Work out the finished part from the listing and answer in its coordinate system (mm). Coordinates: 2 decimals unless noted, no trailing zeros. Order: outer loops, then holes, each group sorted by start corner. A loop starts at its lowest first (then second) coordinate and runs counter-clockwise, first axis right, second up.
1. The part is cut by section A-A, the plane z = 12.7. Give the vertices of the cut face in (x, y).
2. The part is cut by section B-B, the plane z = 0. Give the vertices of the cut face in (x, y), then the cut area to 3 significant figures.
3. Flat-ended cylindrical pins translate along their axes: pin 1 Ø0.6 at (x, y) = (-33, 3) entering from +Z; pin 2 Ø2 at (y, z) = (3.5, 39.5) entering from -X; pin 3 Ø1.5 at (x, y) = (-41, 3.5) entering from -Z. Find the tip coordinate at first contact, or state that the pin passes through.
4. The part is cut by section D-D, the plane y = 3.25. Count the separate pieces of the cut face and the enclosed holes in it, then the cut area to 3 significant figures.
5. The part is cut by section C-C, the plane z = 51. Give the vertices of the cut face in (x, y).
6. Find the intervals of material crossed by probe 1 along X at (y, z) = (0.5, 0.5); probe 2 along Z at (x, y) = (-32, 5); probe 3 along Z at (x, y) = (-20.5, 2.75) (3 decimals), in increasing order.
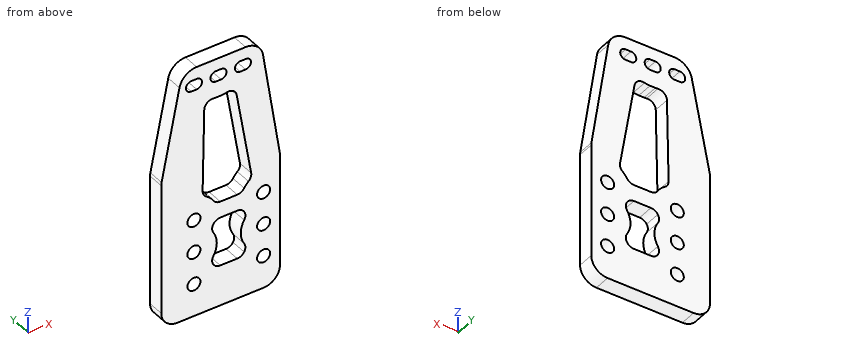
Autodesk Inventor part; units mm, degrees
ref_plane "YZ Plane" through (0, 0, 0) normal (1, 0, 0) x (0, 1, 0)
ref_plane "XZ Plane" through (0, 0, 0) normal (0, 1, 0) x (-1, 0, 0)
ref_plane "XY Plane" through (0, 0, 0) normal (0, 0, 1) x (1, 0, 0)
sketch "Sketch1" plane through (0, 0, 0) normal (0, 1, 0) x (-1, 0, 0)
  line L0 (0, 25.4) -> (0, -25.4) construction
  line L1 (0, -25.4) -> (46.1518, -25.4) construction
  line L2 (15.4178, 64.3509) -> (13.335, 64.3509)
  line L3 (15.4178, 68.5165) -> (13.335, 68.5165)
  arc A0 (13.335, 68.5165) -> (13.335, 64.3509) centre (13.335, 66.4337) ccw
  arc A1 (15.4178, 64.3509) -> (15.4178, 68.5165) centre (15.4178, 66.4337) ccw
  circle A2 centre (13.335, 66.4337) radius 6.8266 construction
  line L4 (32.385, 73.2603) -> (13.335, 73.2603)
  circle A3 centre (6.35, 0) radius 2.54
  circle A4 centre (6.35, -12.7) radius 2.54
  circle A5 centre (6.35, 12.7) radius 2.54
  line L5 (6.35, -12.7) -> (6.35, 12.7) construction
  line L6 (6.5905, 67.4898) -> (0.0764, 25.8882)
  line L7 (0, 24.9059) -> (0, -19.05)
  arc A6 (0.0764, 25.8882) -> (0, 24.9059) centre (6.35, 24.9059) ccw
  line L8 (46.1518, -19.05) -> (46.1518, 31.75)
  line L9 (39.0793, 67.7714) -> (46.0287, 32.9943)
  arc A7 (46.1518, 31.75) -> (46.0287, 32.9943) centre (39.8018, 31.75) ccw
  arc A8 (13.335, 73.2603) -> (6.5905, 67.4898) centre (13.335, 66.4337) ccw
  line L10 (39.8018, -25.4) -> (6.35, -25.4)
  circle A9 centre (33.4518, 12.7) radius 2.54
  circle A10 centre (33.4518, 0) radius 2.54
  circle A11 centre (33.4518, -12.7) radius 2.54
  line L11 (33.4518, -12.7) -> (33.4518, 12.7) construction
  arc A12 (39.8018, -25.4) -> (46.1518, -19.05) centre (39.8018, -19.05) ccw
  arc A13 (0, -19.05) -> (6.35, -25.4) centre (6.35, -19.05) ccw
  arc A14 (24.9428, 64.3509) -> (24.9428, 68.5165) centre (24.9428, 66.4337) ccw
  line L12 (24.9428, 64.3509) -> (22.86, 64.3509)
  line L13 (24.9428, 68.5165) -> (22.86, 68.5165)
  arc A15 (22.86, 68.5165) -> (22.86, 64.3509) centre (22.86, 66.4337) ccw
  circle A16 centre (22.86, 66.4337) radius 6.8266 construction
  arc A17 (34.4678, 64.3509) -> (34.4678, 68.5165) centre (34.4678, 66.4337) ccw
  line L14 (34.4678, 64.3509) -> (32.385, 64.3509)
  line L15 (34.4678, 68.5165) -> (32.385, 68.5165)
  arc A18 (32.385, 68.5165) -> (32.385, 64.3509) centre (32.385, 66.4337) ccw
  circle A19 centre (32.385, 66.4337) radius 6.8266 construction
  arc A20 (39.0793, 67.7714) -> (32.385, 73.2603) centre (32.385, 66.4337) ccw
  line L16 (34.4678, 66.4337) -> (13.335, 66.4337) construction
  point P0 (0, 0)
  point P1 (0, 0)
  point P2 (22.86, 73.2603)
  point P3 (16.1155, 67.4898)
  point P4 (25.6405, 67.4898)
  dimension "d2" = 50.8
  dimension "d3" = 6.35
  dimension "d6" = 91.8337
  dimension "d8" = 13.335
  dimension "d9" = 2.0828
  dimension "d10" = 2.0828
  dimension "d11" = 2.0828
  dimension "d21" = 13.6533
  dimension "d31" = 5.08
  dimension "d32" = 12.7
  dimension "d33" = 12.7
  dimension "d41" = 6.35
  dimension "d42" = 6.35
  dimension "d43" = 13.335
  dimension "d45" = 12.7
  dimension "d46" = 12.7
  dimension "d47" = 6.35
  dimension "d85" = 9.525
  dimension "d90" = 27.1018
extrude "Extrusion3" add sketch "Sketch1" along normal blind 6.35
sketch "Sketch3" plane through (0, 6.35, 0) normal (0, 1, 0) x (1, 0, 0)
  line L0 (-32.385, -73.2603) -> (-13.335, -73.2603) construction
  arc A0 (-13.335, -73.2603) -> (-6.5905, -67.4898) centre (-13.335, -66.4337) ccw construction
  line L1 (-6.5905, -67.4898) -> (-0.0764, -25.8882) construction
  arc A1 (-0.0764, -25.8882) -> (0, -24.9059) centre (-6.35, -24.9059) ccw construction
  line L2 (0, -24.9059) -> (0, 19.05) construction
  arc A2 (0, 19.05) -> (-6.35, 25.4) centre (-6.35, 19.05) ccw construction
  line L3 (-6.35, 25.4) -> (-39.8018, 25.4) construction
  arc A3 (-39.8018, 25.4) -> (-46.1518, 19.05) centre (-39.8018, 19.05) ccw construction
  line L4 (-46.1518, 19.05) -> (-46.1518, -31.75) construction
  arc A4 (-46.1518, -31.75) -> (-46.0287, -32.9943) centre (-39.8018, -31.75) ccw construction
  line L5 (-46.0287, -32.9943) -> (-39.0793, -67.7714) construction
  arc A5 (-39.0793, -67.7714) -> (-32.385, -73.2603) centre (-32.385, -66.4337) ccw construction
  circle A6 centre (-6.35, 0) radius 2.54 construction
  circle A7 centre (-6.35, 12.7) radius 2.54 construction
  circle A8 centre (-6.35, -12.7) radius 2.54 construction
  circle A9 centre (-33.4518, -12.7) radius 2.54 construction
  circle A10 centre (-33.4518, 0) radius 2.54 construction
  circle A11 centre (-33.4518, 12.7) radius 2.54 construction
  line L6 (-34.4678, -64.3509) -> (-32.385, -64.3509) construction
  arc A12 (-32.385, -68.5165) -> (-32.385, -64.3509) centre (-32.385, -66.4337) ccw construction
  line L7 (-32.385, -68.5165) -> (-34.4678, -68.5165) construction
  arc A13 (-34.4678, -64.3509) -> (-34.4678, -68.5165) centre (-34.4678, -66.4337) ccw construction
  line L8 (-24.9428, -64.3509) -> (-22.86, -64.3509) construction
  arc A14 (-22.86, -68.5165) -> (-22.86, -64.3509) centre (-22.86, -66.4337) ccw construction
  line L9 (-22.86, -68.5165) -> (-24.9428, -68.5165) construction
  arc A15 (-24.9428, -64.3509) -> (-24.9428, -68.5165) centre (-24.9428, -66.4337) ccw construction
  arc A16 (-15.4178, -64.3509) -> (-15.4178, -68.5165) centre (-15.4178, -66.4337) ccw construction
  line L10 (-15.4178, -64.3509) -> (-13.335, -64.3509) construction
  arc A17 (-13.335, -68.5165) -> (-13.335, -64.3509) centre (-13.335, -66.4337) ccw construction
  line L11 (-13.335, -68.5165) -> (-15.4178, -68.5165) construction
  line L12 (-32.8524, -66.5271) -> (-39.8018, -31.75) construction
  line L13 (-39.8018, -31.75) -> (-39.8018, 19.05) construction
  line L14 (-39.8018, 19.05) -> (-6.35, 19.05) construction
  line L15 (-6.35, 19.05) -> (-6.35, -24.9059) construction
  line L16 (-6.35, -24.9059) -> (-12.8641, -66.5074) construction
  arc A18 (-13.335, -66.9103) -> (-12.8641, -66.5074) centre (-13.335, -66.4337) ccw construction
  line L17 (-13.335, -66.9103) -> (-32.385, -66.9103) construction
  arc A19 (-32.8524, -66.5271) -> (-32.385, -66.9103) centre (-32.385, -66.4337) ccw construction
  line L18 (-34.4678, -74.8665) -> (-32.385, -74.8665) construction
  arc A20 (-32.385, -74.8665) -> (-32.385, -58.0009) centre (-32.385, -66.4337) ccw construction
  line L19 (-32.385, -58.0009) -> (-34.4678, -58.0009) construction
  arc A21 (-34.4678, -58.0009) -> (-34.4678, -74.8665) centre (-34.4678, -66.4337) ccw construction
  line L20 (-24.9428, -74.8665) -> (-22.86, -74.8665) construction
  arc A22 (-22.86, -74.8665) -> (-22.86, -58.0009) centre (-22.86, -66.4337) ccw construction
  line L21 (-22.86, -58.0009) -> (-24.9428, -58.0009) construction
  arc A23 (-24.9428, -58.0009) -> (-24.9428, -74.8665) centre (-24.9428, -66.4337) ccw construction
  arc A24 (-15.4178, -58.0009) -> (-15.4178, -74.8665) centre (-15.4178, -66.4337) ccw construction
  line L22 (-15.4178, -58.0009) -> (-13.335, -58.0009) construction
  arc A25 (-13.335, -74.8665) -> (-13.335, -58.0009) centre (-13.335, -66.4337) ccw construction
  line L23 (-13.335, -74.8665) -> (-15.4178, -74.8665) construction
  circle A26 centre (-33.4518, -12.7) radius 8.89 construction
  circle A27 centre (-33.4518, 0) radius 8.89 construction
  circle A28 centre (-33.4518, 12.7) radius 8.89 construction
  circle A29 centre (-6.35, 12.7) radius 8.89 construction
  circle A30 centre (-6.35, 0) radius 8.89 construction
  circle A31 centre (-6.35, -12.7) radius 8.89 construction
  line L24 (-24.5618, -12.7) -> (-15.24, -12.7) construction
  line L25 (-24.5618, 12.7) -> (-15.24, 12.7) construction
  line L26 (-32.5524, -58.0009) -> (-33.2753, -21.5882) construction
  line L27 (-13.9947, -58.0009) -> (-7.8293, -21.4661) construction
  line L28 (-29.4371, -54.9642) -> (-30.0738, -22.8937)
  line L29 (-16.8301, -55.7221) -> (-11.1878, -22.2874)
  line L30 (-23.1931, -15.875) -> (-16.6087, -15.875)
  line L31 (-23.1931, -9.525) -> (-16.6087, -9.525)
  line L32 (-23.1931, 9.525) -> (-16.6087, 9.525)
  arc A32 (-28.6237, -20.1647) -> (-25.8927, -17.3789) centre (-33.4518, -12.7) ccw
  arc A33 (-13.9091, -17.3789) -> (-12.2216, -19.3751) centre (-6.35, -12.7) ccw
  arc A34 (-28.6237, -20.1647) -> (-30.0738, -22.8937) centre (-26.8994, -22.8307) ccw
  arc A35 (-23.1931, -15.875) -> (-25.8927, -17.3789) centre (-23.1931, -19.05) ccw
  arc A36 (-13.9091, -17.3789) -> (-16.6087, -15.875) centre (-16.6087, -19.05) ccw
  arc A37 (-11.1878, -22.2874) -> (-12.2216, -19.3751) centre (-14.3185, -21.7591) ccw
  arc A38 (-25.8927, -4.6789) -> (-25.8927, 4.6789) centre (-33.4518, 0) ccw
  arc A39 (-13.9091, 4.6789) -> (-13.9091, -4.6789) centre (-6.35, 0) ccw
  arc A40 (-13.9091, -8.0211) -> (-13.9091, -8.0211) centre (-6.35, -12.7) ccw
  arc A41 (-25.8927, -8.0211) -> (-25.8927, -8.0211) centre (-33.4518, -12.7) ccw
  arc A42 (-25.8927, 8.0211) -> (-25.8927, 8.0211) centre (-33.4518, 12.7) ccw
  arc A43 (-13.9091, 8.0211) -> (-13.9091, 8.0211) centre (-6.35, 12.7) ccw
  arc A44 (-25.8927, -8.0211) -> (-23.1931, -9.525) centre (-23.1931, -6.35) ccw
  arc A45 (-25.8927, -4.6789) -> (-25.8927, -8.0211) centre (-23.1931, -6.35) ccw
  arc A46 (-23.1931, 9.525) -> (-25.8927, 8.0211) centre (-23.1931, 6.35) ccw
  arc A47 (-25.8927, 8.0211) -> (-25.8927, 4.6789) centre (-23.1931, 6.35) ccw
  arc A48 (-13.9091, 8.0211) -> (-16.6087, 9.525) centre (-16.6087, 6.35) ccw
  arc A49 (-13.9091, 4.6789) -> (-13.9091, 8.0211) centre (-16.6087, 6.35) ccw
  arc A50 (-16.6087, -9.525) -> (-13.9091, -8.0211) centre (-16.6087, -6.35) ccw
  arc A51 (-13.9091, -8.0211) -> (-13.9091, -4.6789) centre (-16.6087, -6.35) ccw
  arc A52 (-24.9428, -58.0009) -> (-25.9017, -58.0556) centre (-24.9428, -66.4337) ccw
  arc A53 (-20.7538, -58.2682) -> (-22.86, -58.0009) centre (-22.86, -66.4337) ccw
  arc A54 (-17.2486, -58.202) -> (-19.1389, -58.8663) centre (-15.4178, -66.4337) ccw
  arc A55 (-28.6639, -58.8663) -> (-29.3657, -58.56) centre (-32.385, -66.4337) ccw
  arc A56 (-29.4371, -54.9642) -> (-25.9017, -58.0556) centre (-26.2627, -54.9012) ccw
  arc A57 (-20.7538, -58.2682) -> (-16.8301, -55.7221) centre (-19.9608, -55.1938) ccw
  line L33 (-24.9428, -58.0009) -> (-22.86, -58.0009)
  point P0 (0, 0)
  point P1 (-30.1126, -20.939)
  point P2 (-10.8625, -20.3596)
  point P3 (-25.1481, -15.875)
  point P4 (-14.6537, -15.875)
  point P5 (-25.1481, -9.525)
  point P6 (-14.6537, -9.525)
  point P7 (-25.1481, 9.525)
  point P8 (-14.6537, 9.525)
  point P9 (-13.9091, 8.0211)
  point P10 (-25.8927, 8.0211)
  dimension "d93" = 6.35
  dimension "d94" = 6.35
  dimension "d95" = 6.35
  dimension "d96" = 6.35
  dimension "d97" = 6.35
  dimension "d98" = 6.35
  dimension "d99" = 6.35
  dimension "d100" = 6.35
  dimension "d101" = 6.35
  dimension "d102" = 6.35
  dimension "d104" = 3.175
  dimension "d105" = 3.175
  dimension "d107" = 3.175
  dimension "d108" = 3.175
  dimension "d109" = 3.175
  dimension "d112" = 3.175
  dimension "d113" = 3.175
  dimension "d114" = 3.175
  dimension "d115" = 3.175
  dimension "d116" = 3.175
  dimension "d119" = 3.175
extrude "Extrusion5" cut sketch "Sketch3" against normal blind 25.4 contours L28 A34 A32 A35 L30 A36 A33 A37 L29 A57 A53 L33 A52 A56 | A45 A38 A47 A46 L32 A48 A49 A39 A51 A50 L31 A44
properties part number "ELEV_025_CHAINCLAMP1" material "Steel"
Geometry says:
1. outline: (-46.15, 0) - (-35.99, 0) - (-35.99, 6.35) - (-46.15, 6.35) - close; (-30.91, 0) - (-8.89, 0) - (-8.89, 6.35) - (-30.91, 6.35) - close; (-3.81, 0) - (0, 0) - (0, 6.35) - (-3.81, 6.35) - close
2. outline: (-46.15, 0) - (-35.99, 0) - (-35.99, 6.35) - (-46.15, 6.35) - close; (-30.91, 0) - (-24.56, 0) - (-24.56, 6.35) - (-30.91, 6.35) - close; (-15.24, 0) - (-8.89, 0) - (-8.89, 6.35) - (-15.24, 6.35) - close; (-3.81, 0) - (0, 0) - (0, 6.35) - (-3.81, 6.35) - close
2. area: 169 mm2
3. pin 1: stops at z = 73.25
3. pin 2: stops at x = -44.93
3. pin 3: stops at z = -25.38
4. separate pieces: 1
4. enclosed holes: 11
4. area: 3,130 mm2
5. outline: (-42.43, 0) - (-29.52, 0) - (-29.52, 6.35) - (-42.43, 6.35) - close; (-16.03, 0) - (-4.01, 0) - (-4.01, 6.35) - (-16.03, 6.35) - close
6. probe 1: x = -46.15 to -35.94, -30.96 to -24.58, -15.23 to -8.84, -3.86 to 0
6. probe 2: z = -25.4 to -14.78, -10.62 to -2.08, 2.08 to 10.62, 14.78 to 64.39, 68.48 to 73.26
6. probe 3: z = -25.4 to -9.525, 9.525 to 15.875, 58.323 to 73.26
